Can you work these out from the model? Positions are in its coordinate system, mm. Face numbers are marked on the shaded views. Give positions to 0.01 mm unless a question says otherwise; leave off trailing zeros. Loops run counter-clockwise (first coordinate to the right, second up) from the corner with the lowest first, then second, coordinate; pieces in that order, holes last.
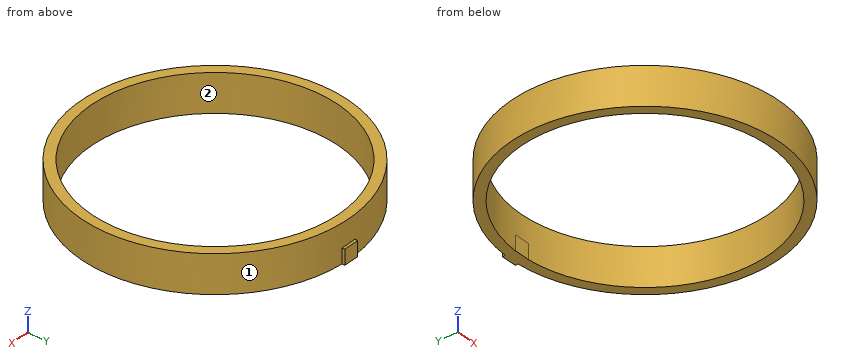
from build123d import *

# Parameters (mm, degrees)
F0_R     = 89.31838
F1_DEPTH = 25.4
F3_D     = 165.1
F3_DEPTH = 101.6
F4_W     = 10.614076
F4_H     = 8.786991
F5_DEPTH = 10


with BuildPart() as f1:
    # F0 (on Top) → F1 (new body)
    with BuildSketch(Plane.XY):
        Circle(F0_R)
    extrude(amount=F1_DEPTH)

    # F3
    with Locations(Plane.XY.offset(25.4)):
        with Locations((0, 0)):
            Hole(F3_D / 2, depth=F3_DEPTH)

    # F4 (on Top) → F5 (join)
    with BuildSketch(Plane.XY):
        with Locations((0, 86.68711)):
            Rectangle(F4_W, F4_H)
    extrude(amount=F5_DEPTH)


solid = f1.part
(1) Suppose I cut it at A-A on x = 0. List the corners of the cut face in (y, z) for me.
Returned:
outline: (-89.32, 0) - (-82.55, 0) - (-82.55, 25.4) - (-89.32, 25.4) - close; (82.29, 0) - (91.08, 0) - (91.08, 10) - (89.32, 10) - (89.32, 25.4) - (82.55, 25.4) - (82.55, 10) - (82.29, 10) - close
(2) Suppose I cut it at C-C on y = -29. List the corners of the cut face in (x, z) for me.
Returned:
outline: (-84.48, 0) - (-77.29, 0) - (-77.29, 25.4) - (-84.48, 25.4) - close; (77.29, 0) - (84.48, 0) - (84.48, 25.4) - (77.29, 25.4) - close
(3) Will these pins go through, and if not, where does the flat tip stop? P1, Ø1.5, axis at x = -52, z = 12.5, coming from the -Y side; P2, Ø12, axis at x = 43, z = 16, coming from the -Y side; P3, Ø2, axis at x = -7.5, z = 12.5, coming from the -Y side; P4, Ø1.5, axis at x = -2, y = 90, coming from the +Z side.
Returned:
P1: stops at y = -73.15
P2: stops at y = -81.29
P3: stops at y = -89.08
P4: stops at z = 25.4
(4) Suppose I cut it at B-B on z = 4.75. List the corners of the cut face in (x, y) for me.
Returned:
outline: (-5.31, 89.16) arc R89.32 ccw (long way) to (5.31, 89.16) - (5.31, 91.08) - (-5.31, 91.08) - close; hole (-5.31, 82.29) - (-5.31, 82.38) arc R82.55 ccw (long way) to (5.31, 82.38) - (5.31, 82.29) - close
(5) Please list where these lines run through material, in increasing order: probe 1 along X at (y, z) = (0, 20.25); probe 2 along Y at (x, z) = (0, 6); probe 3 along X at (y, z) = (-61, 12.5).
Returned:
probe 1: x = -89.32 to -82.55, 82.55 to 89.32
probe 2: y = -89.32 to -82.55, 82.29 to 91.08
probe 3: x = -65.24 to -55.62, 55.62 to 65.24
(6) Suppose I cut it at D-D on y = 45.5. List the corners of the cut face in (x, z) for me.
Returned:
outline: (-76.86, 0) - (-68.88, 0) - (-68.88, 25.4) - (-76.86, 25.4) - close; (68.88, 0) - (76.86, 0) - (76.86, 25.4) - (68.88, 25.4) - close
(7) Thinking about a two-plate mould opening in X: for the marked faces 1 and 2, which applies, pulls with the +X half, pulls with the -X half, needs draft (parallel to the pull), parting line crosses it, or undercut?
Returned:
face 1: parting line crosses it
face 2: undercut
